Geometry check sheet. Reference: drawing and pictorial views, mm from the part's lowest x, y, z. A direction names the side the tool comes from. Give positions to 0.01 mm unless a question says otherwise; leave off trailing zeros. Order: outer loops, then holes, each group sorted by start corner. A loop starts at its lowest first (then second) coordinate and runs counter-clockwise, first axis right, second up. Notation, with made-up numbers: (85.5, 2.25) - (141.5, 2.25) arc R19 ccw to (141.5, 6.25) - close; hole circle Ø11 at (83.5, -3.75). An arc over 180 degrees is marked (long way). Answer in a Markdown table with one row per item.
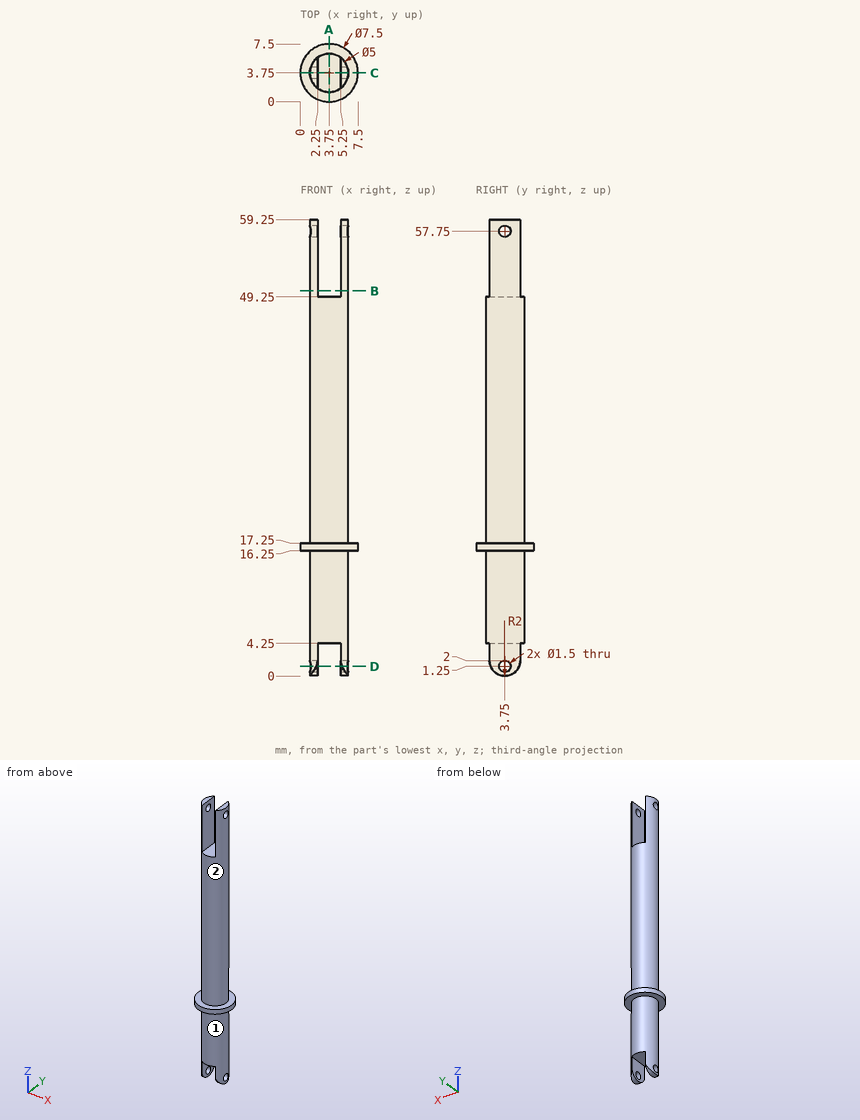
(1) Cross-section at C-C, the plane y = 3.75. Give the number of separate pieces and of enclosed holes in the cut face, then the cut area to 3 significant figures.
Geometry says:
| item | result |
|---|---|
| separate pieces | 5 |
| enclosed holes | 0 |
| area | 250 mm² |
(2) Cross-section at A-A, the plane x = 3.75. Record the cut outline in (y, z).
Geometry says:
| item | result |
|---|---|
| outline | (0, 16.25) - (1.25, 16.25) - (1.25, 4.25) - (6.25, 4.25) - (6.25, 16.25) - (7.5, 16.25) - (7.5, 17.25) - (6.25, 17.25) - (6.25, 49.25) - (1.25, 49.25) - (1.25, 17.25) - (0, 17.25) - close |
(3) Cross-section at B-B, the plane z = 50. Record the cut outline in (x, y), then the cut area to 3 significant figures.
Geometry says:
| item | result |
|---|---|
| outline | (2.25, 1.75) - (2.25, 5.75) arc R2.5 ccw to start; (5.25, 1.75) arc R2.5 ccw to (5.25, 5.75) - close |
| area | 5.59 mm² |
(4) Cross-section at D-D, the plane z = 1.25. Record the cut outline in (x, y), then the cut area to 3 significant figures.
Geometry says:
| item | result |
|---|---|
| outline | (1.37, 3) arc R2.5 ccw to (2.07, 1.9) - (2.25, 1.9) - (2.25, 3) - close; (1.37, 4.5) - (2.25, 4.5) - (2.25, 5.6) - (2.07, 5.6) arc R2.5 ccw to start; (5.25, 1.9) - (5.43, 1.9) arc R2.5 ccw to (6.13, 3) - (5.25, 3) - close; (5.25, 4.5) - (6.13, 4.5) arc R2.5 ccw to (5.43, 5.6) - (5.25, 5.6) - close |
| area | 2.65 mm² |
(5) Gauge pin test, flat ends, axial feed: P1, Ø1.2, axis at y = 4.5, z = 55.5, coming from the -X side; P2, Ø1.4, axis at y = 3.75, z = 57.75, coming from the -X side; P3, Ø2.5, axis at y = 3.75, z = 1.25, coming from the +X side; P4, Ø3.5, axis at x = 4, y = 2.5, coming from the +Z side. Record the tip position at first contact, or that the pin passes through.
Geometry says:
| item | result |
|---|---|
| P1 | x = 1.25 |
| P2 | through |
| P3 | x = 6.25 |
| P4 | z = 59.25 |
(6) Thickness scan on L1, parallel to Z at x = 2, y = 3.75; L2, parallel to Z at x = 2.5, y = 3; L3, parallel to Z at x = 6.5, y = 4.75. Record the ranges inside material, lowest first.
Geometry says:
| item | result |
|---|---|
| L1 | 0 to 0.5, 2 to 57, 58.5 to 59.25 |
| L2 | 4.25 to 49.25 |
| L3 | 16.25 to 17.25 |
(7) Access from +Z, -Z, +X, -X, +Y, -Y to the whole of each face (thin tool, end or side, straight path). Record for the marked faces 1 and 2.
Geometry says:
| item | result |
|---|---|
| face 1 | -Z |
| face 2 | +Z |
